Job drawing, mm, ordinate dimensions from the low corner. One solid piece. A direction names the side the tool comes from. Round coordinates to 2 decimals unless told otherwise and drop trailing zeros. Loops run counter-clockwise (first coordinate to the right, second up) from the corner with the lowest first, then second, coordinate; pieces in that order, holes last.
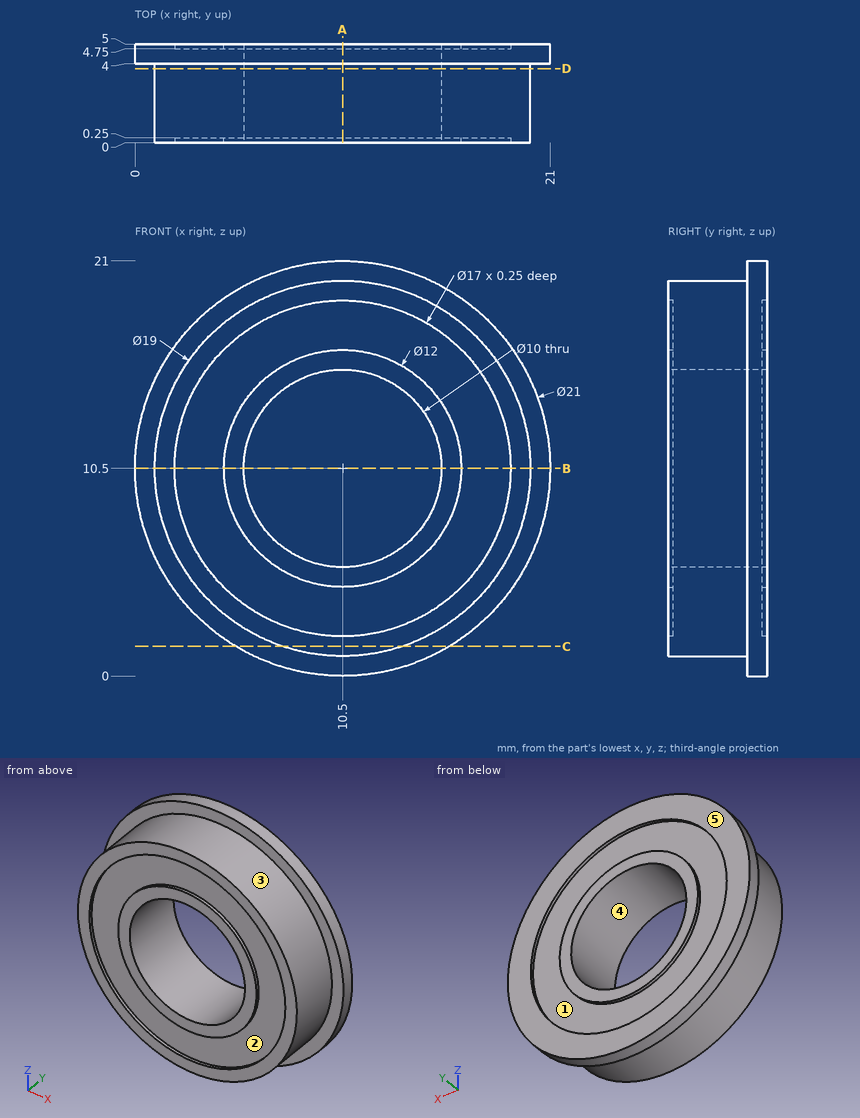
Item 1: Probe line 1 (X direction, y = 0.1, z = 10.5); line 2 (Y direction, x = 12, z = 3); line 3 (Y direction, x = 1.25, z = 13.5). List the from-to ranges inside material, lowest first.
Answers follow:
line 1: x = 1 to 2, 4.5 to 5.5, 15.5 to 16.5, 19 to 20
line 2: y = 0.25 to 4.75
line 3: y = 4 to 5
Item 2: Cut at C-C, the plane z = 1.5. Give the cut face in (x, y), plus the area to 3 significant figures.
Answers follow:
outline: (5.09, 4) - (7.46, 4) - (7.46, 0) - (13.54, 0) - (13.54, 4) - (15.91, 4) - (15.91, 5) - (5.09, 5) - close
area: 35.1 mm2
Item 3: Cut at B-B, the plane z = 10.5. Give the cut face in (x, y).
Answers follow:
outline: (0, 4) - (1, 4) - (1, 0) - (2, 0) - (2, 0.25) - (4.5, 0.25) - (4.5, 0) - (5.5, 0) - (5.5, 5) - (4.5, 5) - (4.5, 4.75) - (2, 4.75) - (2, 5) - (0, 5) - close; (15.5, 0) - (16.5, 0) - (16.5, 0.25) - (19, 0.25) - (19, 0) - (20, 0) - (20, 4) - (21, 4) - (21, 5) - (19, 5) - (19, 4.75) - (16.5, 4.75) - (16.5, 5) - (15.5, 5) - close
Item 4: Cut at D-D, the plane y = 3.75. Give the cut face in (x, z), plus the area to 3 significant figures.
Answers follow:
outline: circle Ø19 at (10.5, 10.5); hole circle Ø10 at (10.5, 10.5)
area: 205 mm2
Item 5: Two-plate mould, pull along Z, no slides. Class the marked faces 3, 4 and 5: released by +Z, released by -Z, zero draft, split by the parting line, or undercut.
Answers follow:
face 3: split by the parting line
face 4: undercut
face 5: zero draft
Item 6: Flat gauge pins, fed straight in: P1, Ø2, axis at x = 3, y = 0.5, coming from the -Z side; P2, Ø1, axis at y = 1.5, z = 15.5, coming from the -X side; P3, Ø1, axis at x = 12, z = 17.5, coming from the +Y side; P4, Ø6, axis at x = 10.5, z = 10.5, coming from the +Y side. Where does each tip first touch, or does it go through?
Answers follow:
P1: stops at z = 3.57
P2: stops at x = 2.13
P3: stops at y = 4.75
P4: passes through
Item 7: Cut at A-A, the plane x = 10.5. Give the cut face in (y, z), plus the area to 3 significant figures.
Answers follow:
outline: (0, 1) - (4, 1) - (4, 0) - (5, 0) - (5, 2) - (4.75, 2) - (4.75, 4.5) - (5, 4.5) - (5, 5.5) - (0, 5.5) - (0, 4.5) - (0.25, 4.5) - (0.25, 2) - (0, 2) - close; (0, 15.5) - (5, 15.5) - (5, 16.5) - (4.75, 16.5) - (4.75, 19) - (5, 19) - (5, 21) - (4, 21) - (4, 20) - (0, 20) - (0, 19) - (0.25, 19) - (0.25, 16.5) - (0, 16.5) - close
area: 44.5 mm2
Item 8: 3-axis set-ups, long thin cutter, end or side, ignore diameter. For the marked faces 1 and 2: which of +Z, -Z, +X, -X, +Y, -Y reach the whole face in a straight line?
Answers follow:
face 1: +Y
face 2: -Y
